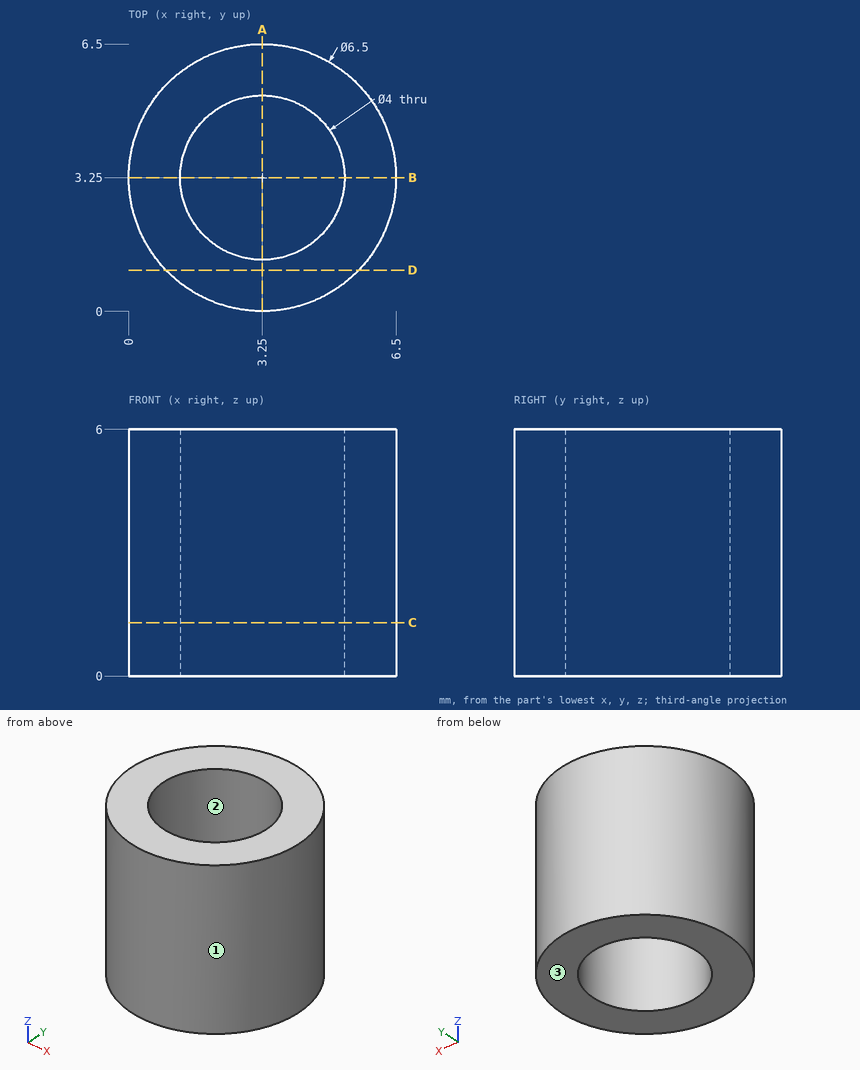
Study the drawing (mm; zero at the part's minimum x, y, z) and answer. Coordinates: 2 decimals unless noted, no trailing zeros. Order: outer loops, then holes, each group sorted by start corner. A loop starts at its lowest first (then second) coordinate and runs counter-clockwise, first axis right, second up. Notation, with made-up numbers: M 4,64 L 62,64 A18 ccw 62,98 Z; hole C 13.5,56 d6. An arc over 180 degrees is marked long. Use CSV: the item, a comma, the result in double quotes.
Q1. Given pin 1 Ø3 at (x, z) = (1.5, 2.5) entering from -Y; pin 2 Ø3.5 at (x, y) = (3.25, 3.25) entering from -Z; pin 3 Ø1.5 at (y, z) = (1.5, 2.5) entering from +X, each flat-ended and moving along its own axis, determine where each tip first touches the part or whether it passes through.
Here are the results:
pin 1,"y = 0.01"
pin 2,"through"
pin 3,"x = 6.34"
Q2. Section A-A (x = 3.25) is taken. Determine the outline of the cut face in (y, z), then the cut area to 3 significant figures.
Here are the results:
outline,"M 0,0 L 1.25,0 L 1.25,6 L 0,6 Z; M 5.25,0 L 6.5,0 L 6.5,6 L 5.25,6 Z"
area,"15.0 mm2"
Q3. Determine the mould class of the marked faces 1, 2 and 3 for opening direction Y: pulls with the +Y half, pulls with the -Y half, needs draft (parallel to the pull), parting line crosses it, or undercut.
Here are the results:
face 1,"parting line crosses it"
face 2,"undercut"
face 3,"needs draft"
Q4. Section C-C (z = 1.3) is taken. Determine the outline of the cut face in (x, y).
Here are the results:
outline,"C 3.25,3.25 d6.5; hole C 3.25,3.25 d4"
Q5. Section D-D (y = 1) is taken. Determine the outline of the cut face in (x, z), then the cut area to 3 significant figures.
Here are the results:
outline,"M 0.9,0 L 5.6,0 L 5.6,6 L 0.9,6 Z"
area,"28.1 mm2"
Q6. Straight lines are drawn through the part: L1, parallel to X at y = 3.25, z = 2.85; L2, parallel to X at y = 1.75, z = 5.3. For each, find the intervals that lie inside material, in ascending order.
Here are the results:
L1,"0 to 1.25, 5.25 to 6.5"
L2,"0.37 to 1.93, 4.57 to 6.13"
